from build123d import *

# Parameters (mm, degrees)
CROQUIS1_W                   = 29
CROQUIS1_H                   = 24
SALIENTE_EXTRUIR1_DEPTH      = 2
CROQUIS2_W                   = 29
CROQUIS2_H                   = 11
CORTAR_EXTRUIR1_DEPTH        = 2
CROQUIS3_R                   = 1.25
CORTAR_EXTRUIR2_DEPTH        = 2
SIMETR_A5_COPY_1_SKETCH_R    = 1.25
SIMETR_A5_COPY_1_DEPTH       = 2
CROQUIS4_W                   = 20
CROQUIS4_H                   = 2
SALIENTE_EXTRUIR2_DEPTH      = 12
CROQUIS6_W                   = 20
CROQUIS6_H                   = 2
SALIENTE_EXTRUIR4_DEPTH      = 12
CROQUIS5_W                   = 20
CROQUIS5_H                   = 2
SALIENTE_EXTRUIR5_DEPTH      = 11
CROQUIS7_R                   = 2.25
CROQUIS7_R_2                 = 1.25
EXTRUIR_L_MINA1_DEPTH        = 7.5
SIMETR_A10_COPY_1_SKETCH_R   = 2.25
SIMETR_A10_COPY_1_SKETCH_R_2 = 1.25
SIMETR_A10_COPY_1_DEPTH      = 7.5
REDONDEO1_R                  = 1.5


with BuildPart() as part:
    # Croquis1 → Saliente-Extruir1 (new body)
    with BuildSketch(Plane.XY):
        Rectangle(CROQUIS1_W, CROQUIS1_H)
    extrude(amount=SALIENTE_EXTRUIR1_DEPTH)

    # Croquis2 → Cortar-Extruir1 (cut)
    with BuildSketch(Plane.XY.offset(2)):
        Rectangle(CROQUIS2_W, CROQUIS2_H)
    extrude(amount=-CORTAR_EXTRUIR1_DEPTH, mode=Mode.SUBTRACT)

    # Croquis3 → Cortar-Extruir2 (cut)
    with BuildSketch(Plane.XY.offset(2)):
        with Locations((-11.5, 9)):
            Circle(CROQUIS3_R)
    cortar_extruir2 = extrude(amount=-CORTAR_EXTRUIR2_DEPTH, mode=Mode.SUBTRACT)

    # Simetría2: Cortar-Extruir2 across plane
    add(cortar_extruir2.mirror(Plane(origin=(0, 0, 0), x_dir=(0, 0, 1), z_dir=(1, 0, 0))), mode=Mode.SUBTRACT)

    # Simetría5: Cortar-Extruir2 across plane
    add(cortar_extruir2.mirror(Plane.ZX), mode=Mode.SUBTRACT)

    # Simetría5 copy 1 sketch → Simetría5 copy 1 (cut)
    with BuildSketch(Plane(origin=(0, 0, 2), x_dir=(-1, 0, 0), z_dir=(0, 0, 1))):
        with Locations((-11.5, 9)):
            Circle(SIMETR_A5_COPY_1_SKETCH_R)
    extrude(amount=-SIMETR_A5_COPY_1_DEPTH, mode=Mode.SUBTRACT)

    # Croquis4 → Saliente-Extruir2 (add)
    with BuildSketch(Plane.XY.offset(2)):
        with Locations((0, 6.5)):
            Rectangle(CROQUIS4_W, CROQUIS4_H)
    extrude(amount=SALIENTE_EXTRUIR2_DEPTH)

    # Croquis6 → Saliente-Extruir4 (add)
    with BuildSketch(Plane.XY.offset(2)):
        with Locations((0, -6.5)):
            Rectangle(CROQUIS6_W, CROQUIS6_H)
    extrude(amount=SALIENTE_EXTRUIR4_DEPTH)

    # Croquis5 → Saliente-Extruir5 (add)
    with BuildSketch(Plane(origin=(0, 5.5, 0), x_dir=(-1, 0, 0), z_dir=(0, -1, 0))):
        with Locations((0, -13)):
            Rectangle(CROQUIS5_W, CROQUIS5_H)
    extrude(amount=SALIENTE_EXTRUIR5_DEPTH)

    # Croquis7 → Extruir-Lámina1 (add)
    with BuildSketch(Plane.XY.offset(2)):
        with Locations((-11.5, 9)):
            Circle(CROQUIS7_R)
        with Locations((-11.5, 9)):
            Circle(CROQUIS7_R_2, mode=Mode.SUBTRACT)
    extruir_l_mina1 = extrude(amount=EXTRUIR_L_MINA1_DEPTH)

    # Simetría8: Extruir-Lámina1 across plane
    add(extruir_l_mina1.mirror(Plane(origin=(0, 0, 0), x_dir=(0, 0, 1), z_dir=(1, 0, 0))))

    # Simetría10: Extruir-Lámina1 across plane
    add(extruir_l_mina1.mirror(Plane.ZX))

    # Simetría10 copy 1 sketch → Simetría10 copy 1 (add)
    with BuildSketch(Plane(origin=(0, 0, 2), x_dir=(-1, 0, 0), z_dir=(0, 0, 1))):
        with Locations((-11.5, 9)):
            Circle(SIMETR_A10_COPY_1_SKETCH_R)
        with Locations((-11.5, 9)):
            Circle(SIMETR_A10_COPY_1_SKETCH_R_2, mode=Mode.SUBTRACT)
    extrude(amount=SIMETR_A10_COPY_1_DEPTH)

    # Redondeo1
    redondeo1_edges = [part.edges().sort_by_distance(p)[0] for p in [
        (10, 6.411474508, 2),
        (-10, -6.411474508, 2),
        (-10, 6.411474508, 2),
        (0, 7.5, 2),
        (10, -6.411474508, 2),
        (0, -7.5, 2),
    ]]
    fillet(redondeo1_edges, radius=REDONDEO1_R)


solid = part.part
For this review, take the finished solid that the model builds, in its own axes (mm). A direction names the side the tool comes from. Give positions to 0.01 mm unless a question says otherwise; leave off trailing zeros. Order: outer loops, then holes, each group sorted by start corner. A loop starts at its lowest first (then second) coordinate and runs counter-clockwise, first axis right, second up. Notation, with made-up numbers: (61, 75.25) -> (102, 75.25) arc R27 cw to (102, 99.25) -> close; hole circle Ø11 at (59, 43). An arc over 180 degrees is marked (long way). Write item = value, one per line.
1) We need section C-C, the plane y = 1. Give the boundary of the cut face in (x, z).
Findings:
outline = (-10, 12) -> (10, 12) -> (10, 14) -> (-10, 14) -> close
2) We need section B-B, the plane x = -6. Give the boundary of the cut face in (y, z), and give its area (3 significant figures).
Findings:
outline = (-12, 0) -> (-5.5, 0) -> (-5.5, 12) -> (5.5, 12) -> (5.5, 0) -> (12, 0) -> (12, 2) -> (9, 2) arc R1.5 cw to (7.5, 3.5) -> (7.5, 14) -> (-7.5, 14) -> (-7.5, 3.5) arc R1.5 cw to (-9, 2) -> (-12, 2) -> close
area = 97.0 mm^2
3) Insertion check: pin 1 (6 mm diameter, centred on y = 9.5, z = 8.5, fed in from -X); pin 2 (3 mm diameter, centred on x = -2.5, y = -10, fed in from +Z); pin 3 (1.5 mm diameter, centred on y = 7, z = 9, fed in from -X). Each pin has a flat end and moves straight along its axis. Give the tip position at first contact, or say it passes through.
Findings:
pin_1 = -13.75
pin_2 = 2.09
pin_3 = -13.37
4) We need section A-A, the plane z = 8.75. Give the boundary of the cut face in (x, y).
Findings:
outline = (-10, -7.32) arc R2.25 ccw (long way) to (-9.82, -7.5) -> (9.82, -7.5) arc R2.25 ccw (long way) to (10, -7.32) -> (10, -5.5) -> (-10, -5.5) -> close; (-10, 5.5) -> (10, 5.5) -> (10, 7.32) arc R2.25 ccw (long way) to (9.82, 7.5) -> (-9.82, 7.5) arc R2.25 ccw (long way) to (-10, 7.32) -> close; hole circle Ø2.5 at (-11.5, -9); hole circle Ø2.5 at (-11.5, 9); hole circle Ø2.5 at (11.5, -9); hole circle Ø2.5 at (11.5, 9)
5) For faces 5 (the face through (0, 9, 0)), 6 (the face through (0, -10, 2)), 7 (the face through (0, 0, 12)), list the 3-axis set-ups (+Z, -Z, +X, -X, +Y, -Y) from which the entire face can be reached by the end or side of a thin tool; tool diameter is ignored.
Findings:
face_5 = -Z, +X, -X, +Y, -Y
face_6 = +Z
face_7 = -Z, +X, -X
6) To check wall thickness, follow L1, parallel to X at y = -9, z = 6.75; L2, parallel to Y at x = 11.5, z = 6; L3, parallel to X at y = -9, z = 1. State the ranges of each line that lie inside material, in increasing order. Write a range as from..to.
Findings:
L1 = -13.75..-12.75, -10.25..-9.25, 9.25..10.25, 12.75..13.75
L2 = -11.25..-10.25, -7.75..-6.75, 6.75..7.75, 10.25..11.25
L3 = -14.5..-12.75, -10.25..10.25, 12.75..14.5
7) Draft analysis for pull direction Y (two halves, no side actions). For faces 1 (the face through (0, -9, 0)), 2 (the face through (0, -12, 1)), 3 (the face through (0, 12, 1)), 4 (the face through (10.43, -6.2, 2.45)), state which applies: pulls with the +Y half, pulls with the -Y half, needs draft (parallel to the pull), parting line crosses it, or undercut.
Findings:
face_1 = needs draft
face_2 = pulls with the -Y half
face_3 = pulls with the +Y half
face_4 = undercut
